from build123d import *

# Parameters (mm, degrees)
BOSS_EXTRUDE1_DEPTH = 1
SKETCH2_R           = 1
CUT_EXTRUDE1_DEPTH  = 10
EXTRUDE_THIN1_START = 0.02
SKETCH3_R           = 2
SKETCH3_R_2         = 1
EXTRUDE_THIN1_DEPTH = 0.02


with BuildPart() as part:
    # Sketch1 → Boss-Extrude1 (new body)
    with BuildSketch(Plane.XY):
        with BuildLine():
            Line((50.5, 52.5), (-30.5, 52.5))
            ThreePointArc((-30.5, 52.5), (-31.914213562, 53.085786438), (-32.5, 54.5))
            Line((-32.5, 54.5), (-32.5, 64.55209468))
            Line((-32.5, 64.55209468), (-50.5, 64.55209468))
            ThreePointArc((-50.5, 64.55209468), (-51.914213562, 63.966308242), (-52.5, 62.55209468))
            Line((-52.5, 62.55209468), (-52.5, 52.5))
            Line((-52.5, 52.5), (-52.5, -52.5))
            Line((-52.5, -52.5), (-52.5, -57.44790532))
            ThreePointArc((-52.5, -57.44790532), (-51.914213562, -58.862118883), (-50.5, -59.44790532))
            Line((-50.5, -59.44790532), (-44.543708146, -59.44790532))
            ThreePointArc((-44.543708146, -59.44790532), (-43.129494584, -60.033691758), (-42.543708146, -61.44790532))
            Line((-42.543708146, -61.44790532), (-42.543708146, -62))
            Line((-42.543708146, -62), (37.456291854, -62))
            Line((37.456291854, -62), (37.456291854, -57.5))
            ThreePointArc((37.456291854, -57.5), (38.920757948, -53.964466094), (42.456291854, -52.5))
            Line((42.456291854, -52.5), (50.5, -52.5))
            ThreePointArc((50.5, -52.5), (51.914213562, -51.914213562), (52.5, -50.5))
            Line((52.5, -50.5), (52.5, 50.5))
            ThreePointArc((52.5, 50.5), (51.914213562, 51.914213562), (50.5, 52.5))
        make_face()
    extrude(amount=BOSS_EXTRUDE1_DEPTH)

    # Sketch2 → Cut-Extrude1 (cut)
    with BuildSketch(Plane.XY.offset(1)):
        with Locations((-41.5, 61.55209468)):
            Circle(SKETCH2_R)
        with Locations((-47.521854073, -56.44790532)):
            Circle(SKETCH2_R)
        with Locations((49.5, 37.474161099)):
            Circle(SKETCH2_R)
        with Locations((46.5, -47.340248832)):
            Circle(SKETCH2_R)
    extrude(amount=-CUT_EXTRUDE1_DEPTH, mode=Mode.SUBTRACT)

    # Sketch3 → Extrude-Thin1 (add)
    # profile 1 of 4: a face of its own
    with BuildSketch(Plane.XY.offset(1).offset(EXTRUDE_THIN1_START)):
        with Locations((-47.521854073, -56.44790532)):
            Circle(SKETCH3_R)
        with Locations((-47.521854073, -56.44790532)):
            Circle(SKETCH3_R_2, mode=Mode.SUBTRACT)
    # profile 2 of 4: a face of its own
    with BuildSketch(Plane.XY.offset(1).offset(EXTRUDE_THIN1_START)):
        with Locations((-41.5, 61.55209468)):
            Circle(SKETCH3_R)
        with Locations((-41.5, 61.55209468)):
            Circle(SKETCH3_R_2, mode=Mode.SUBTRACT)
    # profile 3 of 4: a face of its own
    with BuildSketch(Plane.XY.offset(1).offset(EXTRUDE_THIN1_START)):
        with Locations((49.5, 37.474161099)):
            Circle(SKETCH3_R)
        with Locations((49.5, 37.474161099)):
            Circle(SKETCH3_R_2, mode=Mode.SUBTRACT)
    # profile 4 of 4: a face of its own
    with BuildSketch(Plane.XY.offset(1).offset(EXTRUDE_THIN1_START)):
        with Locations((46.5, -47.340248832)):
            Circle(SKETCH3_R)
        with Locations((46.5, -47.340248832)):
            Circle(SKETCH3_R_2, mode=Mode.SUBTRACT)
    extrude(amount=-EXTRUDE_THIN1_DEPTH)


solid = part.part
Source: CAD feature listing. Evaluate the final solid. Frame: model axes, mm. Round coordinates to 2 decimals unless told otherwise and drop trailing zeros. Order: outer loops, then holes, each group sorted by start corner. A loop starts at its lowest first (then second) coordinate and runs counter-clockwise, first axis right, second up. Notation, with made-up numbers: (-14, 23) -> (-2, 23) arc R8 cw to (-2, 38) -> close; hole circle Ø6 at (21, 76.25). An arc over 180 degrees is marked (long way). Answer as CSV lines item,"result".
Item 1: Section B-B, the plane y = 28. Return loops of the section in (x, z), plus the area to 3 significant figures.
A:
outline,"(-52.5, 0) -> (52.5, 0) -> (52.5, 1) -> (-52.5, 1) -> close"
area,"105 mm²"
Item 2: Pin query (flat end, axial travel): pin 1 Ø1.2 at (x, y) = (49.5, 37.47) entering from -Z; pin 2 Ø0.5 at (x, z) = (2, 0.5) entering from +Y; pin 3 Ø0.5 at (x, z) = (47, 0.5) entering from -Y; pin 4 Ø0.5 at (y, z) = (-60.5, 0.5) entering from +X. Return the tip coordinate at first contact, or that it passes through.
A:
pin 1,"through"
pin 2,"y = 52.5"
pin 3,"y = -52.5"
pin 4,"x = 37.46"
Item 3: Line query: L1, parallel to Y at x = -41.5, z = 0.4; L2, parallel to Z at x = -9, y = -1; L3, parallel to Y at x = -13.5, z = 0.85. Output: solid intervals per line, ascending.
A:
L1,"-62 to 60.55, 62.55 to 64.55"
L2,"0 to 1"
L3,"-62 to 52.5"
Item 4: Section A-A, the plane z = 0.65. Return loops of the section in (x, y).
A:
outline,"(-52.5, -57.45) arc R2 ccw to (-50.5, -59.45) -> (-44.54, -59.45) arc R2 cw to (-42.54, -61.45) -> (-42.54, -62) -> (37.46, -62) -> (37.46, -57.5) arc R5 cw to (42.46, -52.5) -> (50.5, -52.5) arc R2 ccw to (52.5, -50.5) -> (52.5, 50.5) arc R2 ccw to (50.5, 52.5) -> (-30.5, 52.5) arc R2 cw to (-32.5, 54.5) -> (-32.5, 64.55) -> (-50.5, 64.55) arc R2 ccw to (-52.5, 62.55) -> close; hole circle Ø2 at (-47.52, -56.45); hole circle Ø2 at (-41.5, 61.55); hole circle Ø2 at (46.5, -47.34); hole circle Ø2 at (49.5, 37.47)"
Item 5: Section C-C, the plane x = -20. Return loops of the section in (y, z).
A:
outline,"(-62, 0) -> (52.5, 0) -> (52.5, 1) -> (-62, 1) -> close"
